Geometry check sheet. Reference: the model listing, model coordinates, mm. A direction names the side the tool comes from. Round coordinates to 2 decimals unless told otherwise and drop trailing zeros. Loops run counter-clockwise (first coordinate to the right, second up) from the corner with the lowest first, then second, coordinate; pieces in that order, holes last. Notation, with made-up numbers: M 28,35 L 57,35 A19 cw 57,70 Z; hole C 22,27.25 d3. An arc over 180 degrees is marked long. Use one line per item in the form item = value. Start each with the question number.
1. Draft check along Z on faces 1 (the flat face through (3, -2, 12)), 2 (the flat face through (-7, 15, 17)), 3 (the flat face through (-9.46, 30.54, -3.59)). Enter one of: pulls with the +Z half, pulls with the -Z half, needs draft (parallel to the pull), parting line crosses it, or undercut.
2. Cross-section at C-C (y = 17.5). Record the boundary of the cut face in (x, z), then the cut area to 3 significant figures.
3. Set-up check for faces 4 (the flat face through (-1.95, 0, -8)), 5 (the flat face through (-10.24, 0.46, -11.96)), 6 (the flat face through (-9, 15, 0)), 7 (the flat face through (-10.24, 30.54, -11.96)): record each of +Z, -Z, +X, -X, +Y, -Y from which the full face is reachable in a straight line by a thin tool's end or side.
4. Cross-section at A-A (y = 21). Record the boundary of the cut face in (x, z), then the cut area to 3 significant figures.
5. Cross-section at D-D (x = 6). Record the boundary of the cut face in (y, z), then the cut area to 3 significant figures.
6. Material ranges on line 1 (X direction, y = 15, z = 12); line 2 (Y direction, x = 8.5, z = 4); line 3 (Y direction, x = 11.9, z = 3), recorded low to high.
7. Cross-section at B-B (z = 12). Record the boundary of the cut face in (x, y), then the cut area to 4 significant figures.
8. Go/stop test with flat-tipped pins: pin 1 (8 mm diameter, centred on x = -9, z = -5.5, fed in from -Y); pin 2 (1.5 mm diameter, centred on x = 7.5, y = 3.5, fed in from +Z); pin 3 (8 mm diameter, centred on x = -7, z = 12, fed in from -Y); pin 4 (8 mm diameter, centred on x = 6, y = 22.5, fed in from +Z). Record where each tip stops, or that it passes through.
```python
from build123d import *

# Parameters (mm, degrees)
ESQUISSE1_W             = 15
ESQUISSE1_H             = 35
ESQUISSE1_W_2           = 11
ESQUISSE1_H_2           = 31
EXTRU_MINCE1_DEPTH      = 28
ESQUISSE2_W             = 11
ESQUISSE2_H             = 5
BOSS_EXTRU_1_DEPTH      = 14
BOSS_EXTRU_2_REACH      = 48.669
ESQUISSE8_R             = 3.1
ESQUISSE3_R             = 1.6
ESQUISSE3_R_2           = 1.639162694
ENL_V_MAT_EXTRU_1_DEPTH = 50.979995998
ENL_V_MAT_EXTRU_2_DEPTH = 5


with BuildPart() as part:
    # Esquisse1 → Extru.-Mince1 (new body)
    with BuildSketch(Plane.XY):
        with Locations((5.5, 15.5)):
            Rectangle(ESQUISSE1_W, ESQUISSE1_H)
        with Locations((5.5, 15.5)):
            Rectangle(ESQUISSE1_W_2, ESQUISSE1_H_2, mode=Mode.SUBTRACT)
    extrude(amount=EXTRU_MINCE1_DEPTH)

    # Esquisse2 → Boss.-Extru.1 (add)
    with BuildSketch(Plane(origin=(0, 0, 0), x_dir=(-1, 0, 0), z_dir=(0, 0, -1))):
        with Locations((-5.5, 2.5)):
            Rectangle(ESQUISSE2_W, ESQUISSE2_H)
    extrude(amount=-BOSS_EXTRU_1_DEPTH)

    # Boss.-Extru.2: up to this face of the body (flat: up to its plane)
    boss_extru_2_end = Plane(part.part.faces().sort_by_distance((5.5, 33, 14))[0])
    # Esquisse8 → Boss.-Extru.2 (add, up to the picked face)
    with BuildSketch(Plane.XZ.offset(2), mode=Mode.PRIVATE) as boss_extru_2_sk1:
        Polygon((-2, 17), (-12, 17), (-12, 7), (-7, 2), (-12, -3), (-12, -13), (-2, -13), (0, 0), (-2, 0), align=None)
        with Locations(Location((-7, 12, 0), (0, 0, 270))):
            Circle(ESQUISSE8_R, mode=Mode.SUBTRACT)
        with Locations(Location((-7, -8, 0), (0, 0, 270))):
            Circle(ESQUISSE8_R, mode=Mode.SUBTRACT)
    boss_extru_2_tool1 = split(extrude(boss_extru_2_sk1.sketch, amount=-BOSS_EXTRU_2_REACH, mode=Mode.PRIVATE), bisect_by=boss_extru_2_end, keep=Keep.BOTH, mode=Mode.PRIVATE)
    add(boss_extru_2_tool1.solids().sort_by(Axis((-6.31025, -2, 1.638284), (0, 1, 0)))[0])

    # Esquisse3 → Enlèv. mat.-Extru.1 (cut, through all)
    with BuildSketch(Plane(origin=(13, 0, 0), x_dir=(0, 0, -1), z_dir=(1, 0, 0))):
        with Locations(Location((-3, 8, 0), (0, 0, 51.317812547))):
            Circle(ESQUISSE3_R)
        with Locations((-25, 21)):
            Circle(ESQUISSE3_R_2)
    extrude(amount=-ENL_V_MAT_EXTRU_1_DEPTH, mode=Mode.SUBTRACT)

    # Esquisse9 → Enlèv. mat.-Extru.2 (cut)
    with BuildSketch(Plane.XZ.offset(2)):
        Polygon((-7, -2.168762281), (-12.05, -5.084381141), (-12.05, -10.915618859), (-7, -13.831237719), (-1.95, -10.915618859), (-1.95, -5.084381141), align=None)
        Polygon((-1.95, 14.915618859), (-7, 17.831237719), (-12.05, 14.915618859), (-12.05, 9.084381141), (-7, 6.168762281), (-1.95, 9.084381141), align=None)
    enl_v_mat_extru_2 = extrude(amount=-ENL_V_MAT_EXTRU_2_DEPTH, mode=Mode.SUBTRACT)

    # Symétrie1: Enlèv. mat.-Extru.2 across plane
    add(enl_v_mat_extru_2.mirror(Plane(origin=(0, 15.5, 0), x_dir=(0, 0, 1), z_dir=(0, -1, 0))), mode=Mode.SUBTRACT)


solid = part.part
```
Reported:
q1.face_1 = needs draft
q1.face_2 = pulls with the +Z half
q1.face_3 = undercut
q2.outline = M -12,-13 L -2,-13 L 0,0 L 0,28 L -2,28 L -2,17 L -12,17 L -12,7 L -7,2 L -12,-3 Z; M 11,0 L 13,0 L 13,28 L 11,28 Z; hole C -7,-8 d6.2; hole C -7,12 d6.2
q2.area = 340 mm²
q3.face_4 = -X, -Y
q3.face_5 = -Y
q3.face_6 = -X, +Y, -Y
q3.face_7 = +Y
q4.outline = M -12,-13 L -2,-13 L 0,0 L 0,23.36 L -2,23.36 L -2,17 L -12,17 L -12,7 L -7,2 L -12,-3 Z; M -2,26.64 L 0,26.64 L 0,28 L -2,28 Z; M 11,0 L 13,0 L 13,23.36 L 11,23.36 Z; M 11,26.64 L 13,26.64 L 13,28 L 11,28 Z; hole C -7,-8 d6.2; hole C -7,12 d6.2
q4.area = 327 mm²
q5.outline = M -2,0 L 5,0 L 5,14 L 0,14 L 0,28 L -2,28 Z; M 31,0 L 33,0 L 33,28 L 31,28 Z
q5.area = 182 mm²
q6.line_1 = -12 to -10.1, -3.9 to 0, 11 to 13
q6.line_2 = -2 to 5, 31 to 33
q6.line_3 = -2 to 6.4, 9.6 to 33
q7.outline = M -12,3 L -10.1,3 L -10.1,28 L -12,28 Z; M -3.9,3 L -1.95,3 L -1.95,-2 L 13,-2 L 13,33 L -1.95,33 L -1.95,28 L -3.9,28 Z; hole M 0,5 L 11,5 L 11,31 L 0,31 Z
q7.area = 333.5 mm²
q8.pin_1 = -2
q8.pin_2 = 14
q8.pin_3 = 3
q8.pin_4 = through
